from build123d import *

# Parameters (mm, degrees)
F0_R     = 3
F0_R_2   = 4.5
F1_DEPTH = 8


with BuildPart() as f1:
    # F0 (on Front) → F1 (new body)
    with BuildSketch(Plane.XZ):
        with BuildLine():
            ThreePointArc((0, 20.5), (5.3033008589, 22.6966991411), (7.5, 28))
            ThreePointArc((7.5, 28), (6.4388708267, 31.8458994367), (3.5557486728, 34.6035332494))
            ThreePointArc((3.5557486728, 34.6035332494), (-7.2724307962, 29.8335076533), (0, 20.5))
        make_face()
        with Locations((0, 28)):
            Circle(F0_R, mode=Mode.SUBTRACT)
        with BuildLine():
            ThreePointArc((3.5557486728, 34.6035332494), (6.4388708267, 31.8458994367), (7.5, 28))
            ThreePointArc((7.5, 28), (5.3033008589, 22.6966991411), (0, 20.5))
            add(Edge.make_bspline(
                [(0, -20.5), (28.5625234834, -20.5), (28.5625234834, 0), (28.5625234834, 20.5), (0, 20.5)],
                knots=[4.7123889804, 4.7123889804, 4.7123889804, 6.2831853072, 6.2831853072, 7.853981634, 7.853981634, 7.853981634], degree=2, weights=[1, 0.7071067812, 1, 0.7071067812, 1]))
            ThreePointArc((0, -20.5), (5.3033008589, -22.6966991411), (7.5, -28))
            ThreePointArc((7.5, -28), (6.4388708267, -31.8458994367), (3.5557486728, -34.6035332494))
            Line((3.5557486728, -34.6035332494), (55.5557486728, -6.6035332494))
            ThreePointArc((55.5557486728, -6.6035332494), (44.5, 0), (55.5557486728, 6.6035332494))
            Line((55.5557486728, 6.6035332494), (3.5557486728, 34.6035332494))
        make_face()
        with BuildLine():
            ThreePointArc((59.5, 0), (58.4388708267, 3.8458994367), (55.5557486728, 6.6035332494))
            ThreePointArc((55.5557486728, 6.6035332494), (44.5, 0), (55.5557486728, -6.6035332494))
            ThreePointArc((55.5557486728, -6.6035332494), (58.4388708267, -3.8458994367), (59.5, 0))
        make_face()
        with Locations((52, 0)):
            Circle(F0_R_2, mode=Mode.SUBTRACT)
        with BuildLine():
            ThreePointArc((7.5, -28), (5.3033008589, -22.6966991411), (0, -20.5))
            ThreePointArc((0, -20.5), (-7.2724307962, -29.8335076533), (3.5557486728, -34.6035332494))
            ThreePointArc((3.5557486728, -34.6035332494), (6.4388708267, -31.8458994367), (7.5, -28))
        make_face()
        with Locations((0, -28)):
            Circle(F0_R, mode=Mode.SUBTRACT)
    extrude(amount=F1_DEPTH)


solid = f1.part
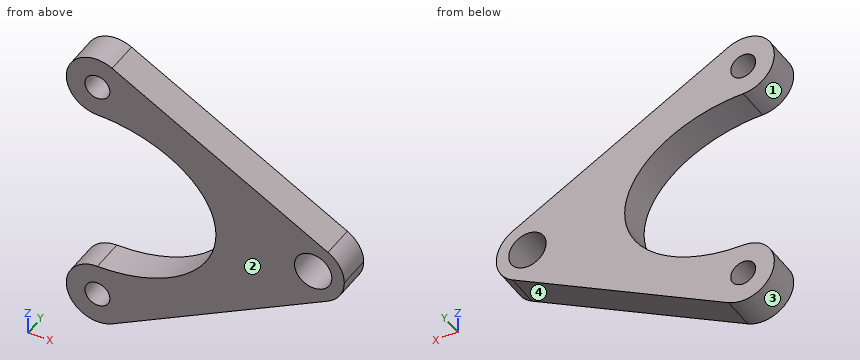
Design review of the part built by this model. Coordinates are the model's own, in mm. Face numbers are marked on the shaded views. Coordinates: 2 decimals unless noted, no trailing zeros. Write each loop counter-clockwise with the first axis right and the second up, starting at its lowest first coordinate (ties: lowest second). Pieces come first, ordered by that corner, then holes. Notation, with made-up numbers: (56, 55) -> (93, 55) arc R19 ccw to (93, 70) -> close; hole circle Ø10 at (59, 48.25). An arc over 180 degrees is marked (long way). Write each question's results on one line, items separated by ' | '. Start each with the question number.
(1) Clearance check with flat-ended pins moving along their axes: P1, Ø3, axis at y = -4, z = -16.5, coming from the +X side; P2, Ø1.5, axis at x = 1, z = 22.5, coming from the +Y side; P3, Ø1, axis at x = 9, y = -6, coming from the -Z side. State where each tip first meets the part, or that it passes through.
(2) Take a section at B-B on x = 53.5. Write out the cut boundary in (y, z).
(3) Take a section at A-A on z = 26.5. Write out the cut boundary in (x, y).
(4) For line 1 along Z through (x, y) = (21, -4.5); line 2 along X through (y, z) = (-5, 26); line 3 along X through (y, z) = (-3.75, -27), list the stretches that pass through material, from the lowest coordinate up. Write a range as from..to.
(5) Take a section at C-C on y = -7. Give the number of separate pieces and of enclosed holes in the cut face, and give its area (3 significant figures).
(6) Take a section at D-D on x = 33.5. Write out the cut boundary in (y, z), and give its area (3 significant figures).
(7) The part is to be moulded in two halves that separate along Z. For the marked faces 1, 2, 3 and 4, say which applies: pulls with the +Z half, pulls with the -Z half, needs draft (parallel to the pull), parting line crosses it, or undercut.
Results found:
1) P1: stops at x = 39.96 | P2: stops at y = 0 | P3: stops at z = -31.94
2) outline: (-8, -7.71) -> (0, -7.71) -> (0, -4.24) -> (-8, -4.24) -> close; (-8, 4.24) -> (0, 4.24) -> (0, 7.71) -> (-8, 7.71) -> close
3) outline: (-7.35, -8) -> (-2.6, -8) -> (-2.6, 0) -> (-7.35, 0) -> close; (2.6, -8) -> (18.61, -8) -> (18.61, 0) -> (2.6, 0) -> close
4) line 1: z = -25.21..-13.9, 13.9..25.21 | line 2: x = -7.23..-2.24, 2.24..19.53 | line 3: x = -7.43..-2.83, 2.83..17.68
5) separate pieces: 1 | enclosed holes: 3 | area: 1,570 mm2
6) outline: (-8, -18.48) -> (0, -18.48) -> (0, 18.48) -> (-8, 18.48) -> close | area: 296 mm2
7) face 1: undercut | face 2: needs draft | face 3: undercut | face 4: pulls with the -Z half
